```python
from build123d import *

# Parameters (mm, degrees)
F0_R     = 11.0998
F1_DEPTH = 6.9342
F2_SIZE  = 3.4671
F3_SIZE  = 3.46709
F5_DEPTH = 6.9342
F6_SIZE  = 3.46709


# Not quite as in the source:
# - a fillet or chamfer is up to 0.001 mm smaller than in the source, because OpenCascade refuses the exact size


with BuildPart() as f1:
    # F0 (on Top) → F1 (new body)
    with BuildSketch(Plane.XY):
        Polygon((12.7, 13.7528510513), (0, 45.72), (-12.7, 13.7528510513), (-45.72, 0), (-12.7, -11.6471489487), (0, -45.72), (12.7, -11.6471489487), (45.72, 0), align=None)
        Circle(F0_R, mode=Mode.SUBTRACT)
    extrude(amount=F1_DEPTH)

    # F2
    f2_edges = [f1.edges().sort_by_distance(p)[0] for p in [
        (6.35, -28.683574, 6.9342),
        (29.21, -5.823574, 6.9342),
        (-29.21, -5.823574, 6.9342),
        (-6.35, 29.736426, 6.9342),
        (-29.21, 6.876426, 6.9342),
        (6.35, 29.736426, 6.9342),
        (29.21, 6.876426, 6.9342),
        (-6.35, -28.683574, 6.9342),
    ]]
    chamfer(f2_edges, length=F2_SIZE)

    # F3 (size 3.4671 in the source; OpenCascade refuses exactly that, so slightly less here)
    f3_edges = [f1.edges().sort_by_distance(p)[0] for p in [
        (6.35, -28.683574, 0),
        (29.21, -5.823574, 0),
        (-29.21, -5.823574, 0),
        (-6.35, -28.683574, 0),
        (6.35, 29.736426, 0),
        (29.21, 6.876426, 0),
        (-29.21, 6.876426, 0),
        (-6.35, 29.736426, 0),
    ]]
    chamfer(f3_edges, length=F3_SIZE)

    # F4 (on face) → F5 (join)
    with BuildSketch(Plane.XY.offset(6.9342)):
        Polygon((-5.3285628953, 22.9169632653), (-28.5960960526, 28.4347391196), (-10.0175652565, 11.1142831944), align=None)
        Polygon((-28.5960960526, 28.4347391196), (-21.7413331227, 6.2313264038), (-10.0175652565, 11.1142831944), align=None)
        Polygon((27.3380211817, 29.6928139905), (5.3285628953, 22.9169632653), (10.0175652565, 11.1142831944), align=None)
        Polygon((27.3380211817, 29.6928139905), (10.0175652565, 11.1142831944), (21.7413331227, 6.2313264038), align=None)
        Polygon((10.0175516395, -8.916864886), (5.5819678365, -20.8171000234), (28.5960824356, -26.2373208112), align=None)
        Polygon((-5.5819678365, -20.8171000234), (-10.0175516395, -8.916864886), (-28.504862756, -26.3346525665), align=None)
        Polygon((-10.0175516395, -8.916864886), (-21.9943219535, -4.6922971158), (-28.504862756, -26.3346525665), align=None)
        Polygon((21.9943219535, -4.6922971158), (10.0175516395, -8.916864886), (28.5960824356, -26.2373208112), align=None)
    extrude(amount=-F5_DEPTH)

    # F6 (size 3.4671 in the source; OpenCascade refuses exactly that, so slightly less here)
    f6_edges = [f1.edges().sort_by_distance(p)[0] for p in [
        (17.089025, -23.52721, 6.9342),
        (25.295202, -15.464809, 6.9342),
        (24.539677, 17.96207, 6.9342),
        (-17.043415, -23.575876, 6.9342),
        (-25.249592, -15.513475, 6.9342),
        (-25.168715, 17.333033, 6.9342),
        (-16.962329, 25.675851, 6.9342),
        (16.333292, 26.304889, 6.9342),
        (24.539678, 17.962075, 0),
        (25.295204, -15.464814, 0),
        (17.08903, -23.527212, 0),
        (-17.04342, -23.575877, 0),
        (16.333297, 26.30489, 0),
        (-16.962334, 25.675852, 0),
        (-25.168716, 17.333038, 0),
        (-25.249594, -15.51348, 0),
    ]]
    chamfer(f6_edges, length=F6_SIZE)


solid = f1.part
```
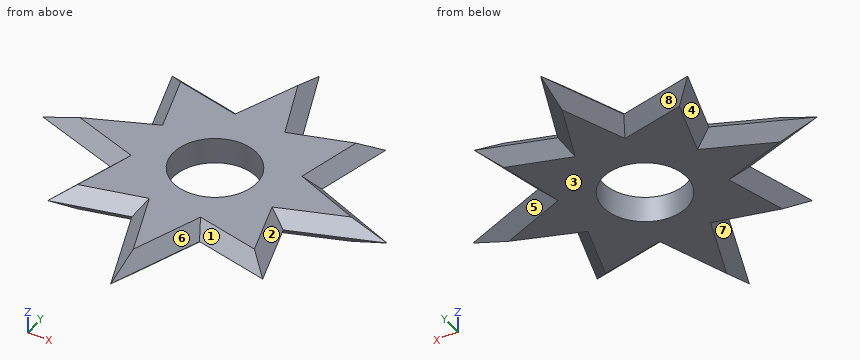
The model under review builds one solid part; all positions refer to its coordinate system, in mm. Face numbers are marked on the shaded views. A direction names the side the tool comes from. Round coordinates to 2 decimals unless told otherwise and drop trailing zeros. Order: outer loops, then holes, each group sorted by start corner. A loop starts at its lowest first (then second) coordinate and runs counter-clockwise, first axis right, second up. Notation, with made-up numbers: (-14, 58.25) -> (-10, 58.25) arc R27 cw to (-10, 88.25) -> close; hole circle Ø6 at (51, 55). An arc over 180 degrees is marked (long way). Use a Markdown table: item, result.
Q1. Clearance check with flat-ended pins moving along their axes: P1, Ø2, axis at x = 18.5, z = 3, coming from the -Y side; P2, Ø4, axis at x = 18.5, y = 25.5, coming from the -Z side. State where each tip first meets the part, or that it passes through.
Values:
| item | result |
|---|---|
| P1 | stops at y = -24.07 |
| P2 | stops at z = 0.06 |
Q2. For line 1 (Y direction, x = -8.5, z = 5.5); line 2 (Y direction, x = 9.5, z = 1.25); line 3 (Y direction, x = -28, z = 6.5), list the stretches that pass through material, from the lowest coordinate up.
Values:
| item | result |
|---|---|
| line 1 | y = -19.43 to -7.14, 7.14 to 21.58 |
| line 2 | y = -19.46 to -5.74, 5.74 to 21.88 |
| line 3 | y = -3.03 to 4.09 |
Q3. Tool access review of the marked faces 4, 5, 6, 7 and 8: name each direction out of +Z, -Z, +X, -X, +Y, -Y from which nothing blocks a thin tool from reaching the whole face with its end or side.
Values:
| item | result |
|---|---|
| face 4 | -Z, -X |
| face 5 | -Z, +X |
| face 6 | +Z, -Y |
| face 7 | -Z, -Y |
| face 8 | -Z, +Y |
Q4. We need section B-B on z = 2.25. Write out the cut boundary in (x, y).
Values:
| item | result |
|---|---|
| outline | (-42.33, 0.09) -> (-21.49, -7.25) -> (-26.73, -24.66) -> (-8.21, -20.2) -> (0, -42.24) -> (8.22, -20.19) -> (26.81, -24.57) -> (21.51, -7.25) -> (42.33, 0.09) -> (21.13, 8.92) -> (25.66, 27.9) -> (7.94, 22.45) -> (0, 42.42) -> (-8, 22.3) -> (-26.81, 26.76) -> (-21.28, 8.86) -> close; hole circle Ø22.2 at (0, 0) |
Q5. Mouldability with a two-part tool opening along X and no side actions: class the marked faces 1, 2 and 3 as +X half, -X half, draft (parallel to the pull), parting line (faces both ways), or undercut.
Values:
| item | result |
|---|---|
| face 1 | undercut |
| face 2 | +X half |
| face 3 | draft |
